Read the model definition and answer for the solid it produces. Units are mm, in the model's axes. Face numbers are marked on the shaded views. A direction names the side the tool comes from. Round coordinates to 2 decimals unless told otherwise and drop trailing zeros. Write each loop counter-clockwise with the first axis right and the second up, starting at its lowest first coordinate (ties: lowest second). Pieces come first, ordered by that corner, then holes.
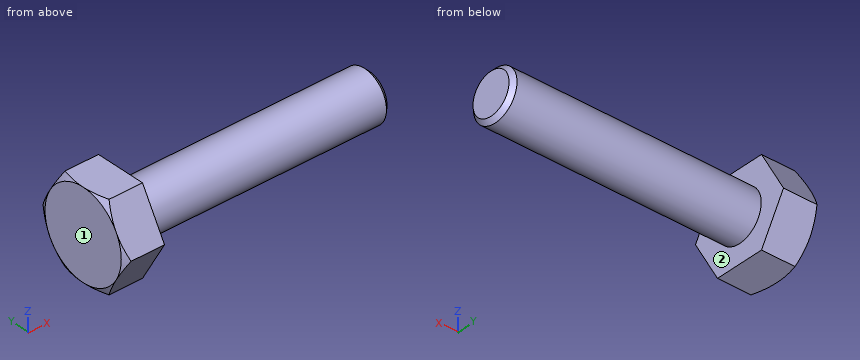
from build123d import *

# Parameters (mm, degrees)
BASEHEAD_DEPTH = 4.7752


with BuildPart() as part:
    # Sketch1 → BaseHead (new body)
    with BuildSketch(Plane(origin=(0, 0, 0), x_dir=(0, 0, -1), z_dir=(1, 0, 0))):
        Polygon((5.5626, 3.211568607), (5.5626, -3.211568607), (0, -6.423137215), (-5.5626, -3.211568607), (-5.5626, 3.211568607), (0, 6.423137215), align=None)
    extrude(amount=BASEHEAD_DEPTH)

    # BodySke → BaseBody (revolve)
    with BuildSketch(Plane.XY):
        Polygon((0, 0), (36.5252, 0), (36.5252, 2.63398), (35.98418, 3.175), (0, 3.175), align=None)
    revolve(axis=Axis((0, 0, 0), (1, 0, 0)))

    # Sketch3 → HeadChamfer (revolve, cut)
    with BuildSketch(Plane.XY):
        Polygon((0, 5.5626), (4.163005602, 12.773137215), (4.163005602, 19.123137215), (-12.7, 19.123137215), (-12.7, 5.5626), align=None)
    revolve(axis=Axis((0, 0, 0), (1, 0, 0)), mode=Mode.SUBTRACT)


solid = part.part
Q1. Straight lines are drawn through the part: probe 1 along X at (y, z) = (3.75, -2.5); probe 2 along Y at (x, z) = (28.5, -2); probe 3 along Z at (x, y) = (21.5, -0.5). For each, find the intervals that lie inside material, in ascending order.
Verdict:
probe 1: x = 0 to 4.78
probe 2: y = -2.47 to 2.47
probe 3: z = -3.14 to 3.14
Q2. Which of the six approach directions +Z, -Z, +X, -X, +Y, -Y give full straight-line access (tool end or side, diameter ignored) to the marked faces 1 and 2?
Verdict:
face 1: +Z, -Z, -X, +Y, -Y
face 2: +X
Q3. Flat-ended cylindrical pins translate along their axes: pin 1 Ø1.5 at (x, y) = (26.5, 5) entering from -Z; pin 2 Ø1 at (x, y) = (5, -2) entering from +Z; pin 3 Ø3 at (x, z) = (30, -2) entering from +Y; pin 4 Ø3 at (x, y) = (25.5, 0.5) entering from +Z (3 decimals). Find the tip coordinate at first contact, or state that the pin passes through.
Verdict:
pin 1: passes through
pin 2: stops at z = 5.56
pin 3: stops at y = 3.14
pin 4: stops at z = 3.175
Q4. Section A-A (x = 28) is taken. Determine the outline of the cut face in (y, z) (3 decimals).
Verdict:
outline: circle Ø6.35 at (0, 0)
